Here's how the part is built. I have some questions about the finished solid (model axes, mm). A direction names the side the tool comes from. Round coordinates to 2 decimals unless told otherwise and drop trailing zeros. Loops run counter-clockwise (first coordinate to the right, second up) from the corner with the lowest first, then second, coordinate; pieces in that order, holes last. Notation, with made-up numbers: M -14.5,10.5 L 17.5,10.5 A29 cw 17.5,39.5 Z; hole C 80.25,80.5 d5. An arc over 180 degrees is marked long. Answer as CSV lines item,"result".
Autodesk Inventor part; units mm, degrees
ref_plane "YZ Plane" through (0, 0, 0) normal (1, 0, 0) x (0, 1, 0)
ref_plane "XZ Plane" through (0, 0, 0) normal (0, 1, 0) x (-1, 0, 0)
ref_plane "XY Plane" through (0, 0, 0) normal (0, 0, 1) x (1, 0, 0)
sketch "Sketch1" plane through (0, 0, 0) normal (0, 0, 1) x (1, 0, 0)
  circle A0 centre (4.5902, 12.1566) radius 1.27
  circle A1 centre (4.5902, -12.1619) radius 1.27
  circle A2 centre (-12.9763, 0.0036) radius 1.27
  line L0 (18.2524, -4.1824) -> (18.2524, 4.1791)
  arc A3 (18.2524, 4.1791) -> (-7.4923, 7.6236) centre (4.5902, -0.0017) ccw
  line L1 (-7.4923, 7.6236) -> (-16.1513, 7.6236)
  line L2 (-16.1513, 7.6236) -> (-16.1513, -7.6164)
  line L3 (-16.1513, -7.6164) -> (-7.4989, -7.6164)
  arc A4 (-7.4989, -7.6164) -> (18.2524, -4.1824) centre (4.5902, -0.0017) ccw
  line L4 (-4.9271, -3.1767) -> (-8.2305, -3.1767)
  arc A5 (-8.2305, 3.1733) -> (-8.2305, -3.1767) centre (4.5902, -0.0017) ccw
  line L5 (-8.2305, 3.1733) -> (-4.9271, 3.1733)
  arc A6 (-4.9271, -3.1767) -> (-4.9271, 3.1733) centre (4.5902, -0.0017) ccw
  circle A7 centre (4.5902, -0.0017) radius 3.175
  circle A8 centre (4.5902, -0.0017) radius 9.017
  circle A9 centre (4.5902, -0.0017) radius 4.953
  point P0 (0, 0)
  dimension "d0" = 1.778
  dimension "d1" = 1.016
extrude "Extrusion1" add sketch "Sketch1" against normal blind 19.05 contours A8
sketch "Sketch2" plane through (4.5902, -0.0017, 0) normal (0, 0, 1) x (1, 0, 0)
  circle A0 centre (0, 0) radius 4.953
  point P0 (-4.5902, 0.0017)
extrude "Extrusion2" add sketch "Sketch2" against normal blind 7.62
sketch "Sketch3" plane through (0, 0, 0) normal (1, 0, 0) x (0, 1, 0)
  line L0 (3.1733, -8.4292) -> (-3.1767, -8.4292)
  point P0 (0, 0)
sketch "Sketch5" plane through (4.5902, -0.0017, 0) normal (0, 0, 1) x (1, 0, 0)
  circle A0 centre (0, 12.1583) radius 1.27
  circle A1 centre (0, -12.1603) radius 1.27
  circle A2 centre (-17.5665, 0.0053) radius 1.27
  line L0 (13.6621, -4.1808) -> (13.6621, 4.1808)
  arc A3 (13.6621, 4.1808) -> (-12.0826, 7.6253) centre (0, 0) ccw
  line L1 (-12.0826, 7.6253) -> (-20.7415, 7.6253)
  line L2 (-20.7415, 7.6253) -> (-20.7415, -7.6147)
  line L3 (-20.7415, -7.6147) -> (-12.0892, -7.6147)
  arc A4 (-12.0892, -7.6147) -> (13.6621, -4.1808) centre (0, 0) ccw
  line L4 (-9.5174, -3.175) -> (-12.8207, -3.175)
  arc A5 (-12.8207, 3.175) -> (-12.8207, -3.175) centre (0, 0) ccw
  line L5 (-12.8207, 3.175) -> (-9.5174, 3.175)
  arc A6 (-9.5174, -3.175) -> (-9.5174, 3.175) centre (0, 0) ccw
  point P0 (-4.5902, 0.0017)
extrude "Extrusion4" add sketch "Sketch5" along normal blind 1.5875 contours A4 L3 L2 L1 A3 L0 | L4 A5 L5 A6
sketch "Sketch6" plane through (4.5902, -0.0017, 1.5875) normal (0, 0, 1) x (1, 0, 0)
  circle A0 centre (0, -12.1603) radius 1.27
  circle A1 centre (0, -12.1603) radius 1.524
  circle A2 centre (-17.5665, 0.0053) radius 1.27
  circle A3 centre (-17.5665, 0.0053) radius 1.524
  circle A4 centre (0, 12.1583) radius 1.27
  circle A5 centre (0, 12.1583) radius 1.524
  point P0 (-4.5902, 0.0017)
  dimension "d12" = 3.048
extrude "Extrusion5" cut sketch "Sketch6" against normal blind 1.5875
sketch "Sketch7" plane through (4.5902, -0.0017, -7.62) normal (0, 0, -1) x (-1, 0, 0)
  circle A0 centre (0, 0) radius 3.429
  point P0 (4.5902, 0.0017)
  dimension "d15" = 6.858
extrude "Extrusion6" cut sketch "Sketch7" against normal up to surface (7.62 mm away)
sketch "Sketch8" plane through (0, 0, 0) normal (0, 1, 0) x (-1, 0, 0)
  spline S0 degree 3 poles (-8.0192, -14.5252) (-8.0192, -14.0929) (-7.9325, -13.6329) (-7.5821, -12.7886) (-7.3185, -12.4041) (-6.7114, -11.797) (-6.3268, -11.5333) (-5.4824, -11.1829) (-5.0225, -11.0962) (-4.158, -11.0962) (-3.698, -11.1829) (-2.8537, -11.5333) (-2.4691, -11.797) (-1.862, -12.4041) (-1.5984, -12.7886) (-1.248, -13.6329) (-1.1612, -14.0929) (-1.1612, -14.9574) (-1.248, -15.4174) (-1.5984, -16.2617) (-1.862, -16.6463) (-2.4691, -17.2534) (-2.8537, -17.517) (-3.698, -17.8675) (-4.158, -17.9542) (-5.0225, -17.9542) (-5.4824, -17.8675) (-6.3268, -17.517) (-6.7114, -17.2534) (-7.3185, -16.6463) (-7.5821, -16.2617) (-7.9325, -15.4174) (-8.0192, -14.9574) (-8.0192, -14.5252) knots 0 0 0 0 0.129682 0.129682 0.259363 0.259363 0.389031 0.389031 0.5187 0.5187 0.648368 0.648368 0.778036 0.778036 0.907718 0.907718 1.037399 1.037399 1.167081 1.167081 1.296762 1.296762 1.426431 1.426431 1.556099 1.556099 1.685767 1.685767 1.815435 1.815435 1.945117 1.945117 2.074799 2.074799 2.074799 2.074799
  point P0 (0, 0)
  point P1 (-8.0192, -14.5252)
extrude "Extrusion7" cut sketch "Sketch8" against normal blind 25.4
sketch "Sketch9" plane through (0, 0, 0) normal (1, 0, 0) x (0, 1, 0)
  line L0 (6.3536, -8.255) -> (-6.3464, -8.255)
  line L1 (-5.4574, -16.7982) -> (5.4646, -16.7982)
  line L2 (5.4646, -8.255) -> (5.4646, -66.0222)
  line L3 (-5.4574, -66.0222) -> (-5.4574, -8.255)
  line L4 (4.9513, -7.62) -> (4.9513, -19.05)
  line L5 (4.9513, -8.255) -> (-5.4574, -8.255)
  line L6 (-5.4574, -8.255) -> (-5.4574, -16.7982)
  line L7 (-5.4574, -16.7982) -> (4.9513, -16.7982)
  line L8 (4.9513, -16.7982) -> (4.9513, -8.255)
  line L9 (4.0885, -8.255) -> (-4.122, -8.255)
  line L10 (-4.122, -8.255) -> (-4.122, -14.2031)
  line L11 (-4.122, -14.2031) -> (4.0885, -14.2031)
  line L12 (4.0885, -14.2031) -> (4.0885, -8.255)
  line L13 (3.81, -8.255) -> (-3.81, -8.255)
  line L14 (-3.81, -8.255) -> (-3.81, -14.605)
  line L15 (-3.81, -14.605) -> (3.81, -14.605)
  line L16 (3.81, -14.605) -> (3.81, -8.255)
  point P0 (0, 0)
  point P1 (0, -14.605)
  dimension "d22" = 6.35
  dimension "d23" = 7.62
extrude "Extrusion8" cut sketch "Sketch9" along normal mid plane 12.7 contours L16 L11 L14 L0 | L16 L15 L14 L11
sketch "Sketch10" plane through (4.5902, -0.0017, 1.5875) normal (0, 0, 1) x (1, 0, 0)
  circle A0 centre (0, 0) radius 3.429
  circle A1 centre (0, 0) radius 2.2479
  point P0 (-4.5902, 0.0017)
  dimension "d24" = 4.4958
extrude "Extrusion9" cut sketch "Sketch10" against normal blind 25.4 contours A1
sketch "Sketch11" plane through (4.5902, -0.0017, -7.62) normal (0, 0, -1) x (-1, 0, 0)
  circle A0 centre (0, 0) radius 4.953
  point P0 (4.5902, 0.0017)
extrude "Extrusion10" cut sketch "Sketch11" against normal blind 3.81
sketch "Sketch12" plane through (4.5902, -0.0017, -19.05) normal (0, 0, -1) x (-1, 0, 0)
  circle A0 centre (0, 0) radius 2.2479
  circle A1 centre (0, 0) radius 36.9649
  point P0 (4.5902, 0.0017)
extrude "Extrusion11" cut sketch "Sketch12" against normal up to surface (15.24 mm away)
sketch "Sketch13" plane through (4.5902, -0.0017, -3.81) normal (0, 0, -1) x (-1, 0, 0)
  circle A0 centre (6.3764, 0.0017) radius 1.5875
  point P0 (4.5902, 0.0017)
  dimension "d31" = 3.175
extrude "Extrusion12" cut sketch "Sketch13" against normal blind 25.4
pattern_circular "Circular Pattern1" count 8 over 360 about axis through (4.5902, -0.0017, 1.5875) along (0, 0, -1) of "Extrusion12"
properties part number "Small Heater Holder for Use With Fan"
1. We'd pull the mould along X, two halves only. Please class faces 4 (the flat face through (18.252, 0, 1)), 5 (the cylindrical face through (0.29, 2.934, -1.149)), 6 (the cylindrical face through (6.258, 14.188, 0.783)), 7 (the flat face through (-12, 7.624, 1)): pulls with the +X half, pulls with the -X half, needs draft (parallel to the pull), parting line crosses it, or undercut.
Evaluation:
face 4,"pulls with the +X half"
face 5,"undercut"
face 6,"parting line crosses it"
face 7,"needs draft"
2. I want a section at B-B, the plane y = 1. Please give me the cut outline in (x, z), and give its area (3 significant figures).
Evaluation:
outline,"M -16.15,0 L -14.13,0 L -14.13,1.59 L -16.15,1.59 Z; M -11.82,0 L -4.37,0 L -4.37,-3.81 L -3.02,-3.81 L -3.02,1.59 L -11.82,1.59 Z; M -0.55,-3.81 L 1.31,-3.81 L 1.31,0 L 2.58,0 L 2.58,1.59 L -0.55,1.59 Z; M 6.6,0 L 7.87,0 L 7.87,-3.81 L 9.74,-3.81 L 9.74,1.59 L 6.6,1.59 Z; M 12.2,-3.81 L 13.55,-3.81 L 13.55,0 L 18.25,0 L 18.25,1.59 L 12.2,1.59 Z"
area,"61.3 mm²"
3. If I drill on line 1 (X direction, y = 0.25, z = -2.1); line 2 (X direction, y = 0.5, z = -3.45); line 3 (Y direction, x = 5.5, z = 0.9), over which ranges is the centre line in solid material (lowest first)? Write a range as [from, to].
Evaluation:
line 1,"x = [-4.42, -3.35], [-0.22, 1.17], [8.01, 9.4], [12.53, 13.6]"
line 2,"x = [-4.41, -3.29], [-0.28, 1.2], [7.98, 9.46], [12.47, 13.59]"
line 3,"y = [-14.26, -13.38], [-10.94, -7.68], [-5.08, -2.06], [2.05, 5.07], [7.68, 10.93], [13.38, 14.26]"
4. Which directions (+Z, -Z, +X, -X, +Y, -Y) give clear straight access to the entire face, cutting with the end or side of a thin tool? Please do faces 1 (the cylindrical face through (4.26, 10.67, 0.8)), 2 (the cylindrical face through (2.635, -8.804, -1.878)), 3 (the flat face through (-12, -7.616, 1)).
Evaluation:
face 1,"+Z, -Z"
face 2,"-Z"
face 3,"+Z, -Z, -X, -Y"
5. I want a section at C-C, the plane z = -0.6. Count the separate pieces of the cut face and the enclosed holes in it, and give its area (3 significant figures).
Evaluation:
separate pieces,"1"
enclosed holes,"9"
area,"155 mm²"
6. For P1, Ø1.7, axis at x = -12, z = 0.5, coming from the -Y side; P2, Ø5, axis at x = 4.59, y = 0, coming from the -Z side; P3, Ø1.5, axis at y = -6.5, z = 0, coming from the +X side; P4, Ø2.5, axis at x = 0.08, y = 4.51, coming from the +Z side, each with a flat end and sliding along its axis, tell me the tip position at first contact or that it passes through.
Evaluation:
P1,"stops at y = -7.62"
P2,"stops at z = 0"
P3,"stops at x = 17.67"
P4,"passes through"
7. I want a section at A-A, the plane x = -14. Please give me the cut outline in (y, z), and give its area (3 significant figures).
Evaluation:
outline,"M -7.62,0 L -1.13,0 L -1.13,1.59 L -7.62,1.59 Z; M 1.13,0 L 7.62,0 L 7.62,1.59 L 1.13,1.59 Z"
area,"20.6 mm²"
8. I want a section at D-D, the plane y = 11. Please give me the cut outline in (x, z).
Evaluation:
outline,"M -4.53,0 L 3.6,0 L 3.6,1.59 L -4.53,1.59 Z; M 5.58,0 L 13.71,0 L 13.71,1.59 L 5.58,1.59 Z"
